Answer from the drawing. Dimensions are ordinates in mm from the lowest x, y and z of the part. A direction names the side the tool comes from. Coordinates: 2 decimals unless noted, no trailing zeros. Write each loop counter-clockwise with the first axis right and the second up, starting at its lowest first coordinate (ties: lowest second). Pieces come first, ordered by that corner, then holes. Notation, with made-up numbers: (-4.5, 62.25) -> (42.5, 62.25) arc R13 ccw to (42.5, 80.25) -> close; hole circle Ø4 at (41.25, 72.25). An arc over 180 degrees is marked (long way). Answer as a JSON object with one key per item and string values. Group by question number.
(1) A straight line is drawn through the part: L1, parallel to X at y = 14, z = 36.5. Find the intervals that lie inside material, in ascending order.
(2) For a pull along Y with two mould halves and no side action, classify the marked faces 1, 2 and 3 as +Y half, -Y half, draft (parallel to the pull), parting line (faces both ways), or undercut.
(3) Find section A-A (x = 11.75). Give the vertices of the cut face in (y, z), then the cut area to 3 significant figures.
(4) Find section C-C (z = 50.5). Give the vertices of the cut face in (x, y).
(5) Which of the six approach directions +Z, -Z, +X, -X, +Y, -Y give full straight-line access (tool end or side, diameter ignored) to the marked faces 4 and 5?
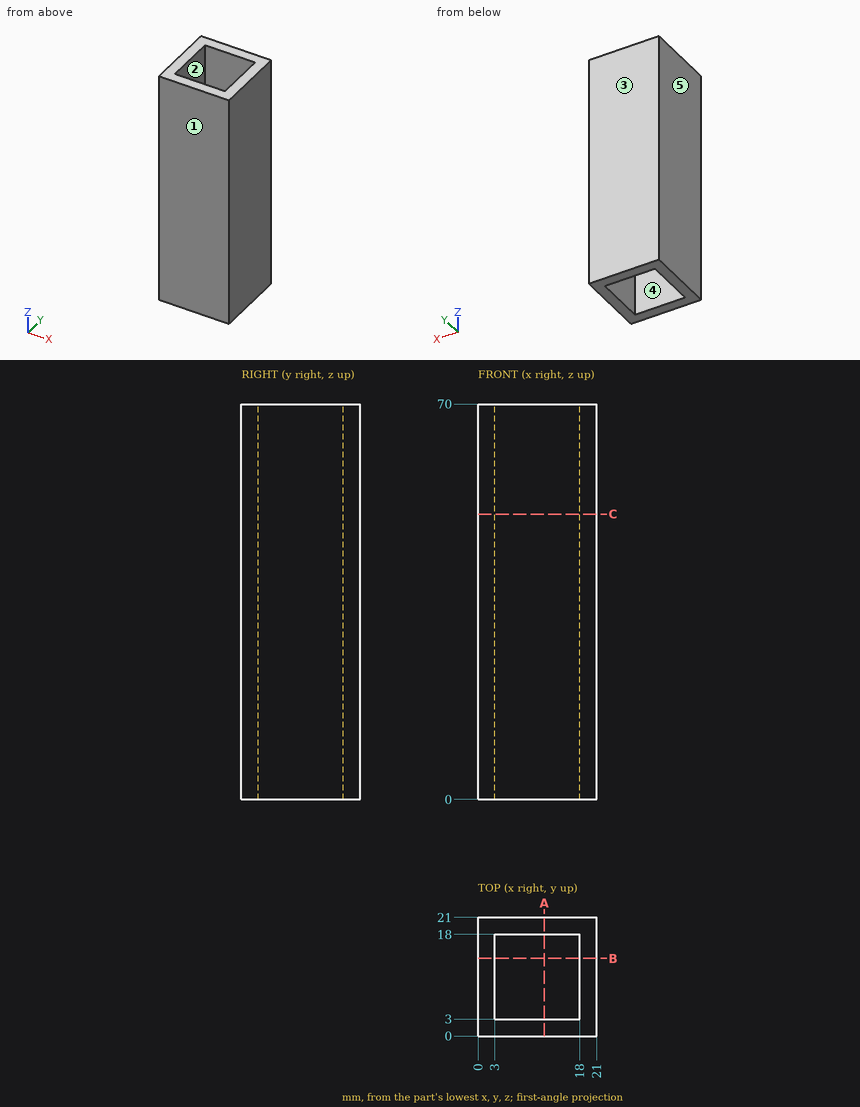
Results below:
{
 "1": {"L1": "x = 0 to 3, 18 to 21"},
 "2": {"face 1": "-Y half", "face 2": "undercut", "face 3": "+Y half"},
 "3": {"outline": "(0, 0) -> (3, 0) -> (3, 70) -> (0, 70) -> close; (18, 0) -> (21, 0) -> (21, 70) -> (18, 70) -> close", "area": "420 mm2"},
 "4": {"outline": "(0, 0) -> (21, 0) -> (21, 21) -> (0, 21) -> close; hole (3, 3) -> (18, 3) -> (18, 18) -> (3, 18) -> close"},
 "5": {"face 4": "+Z, -Z", "face 5": "+Z, -Z, -X, +Y, -Y"}
}
